```python
from build123d import *

# Parameters (mm, degrees)
F0_R     = 2
F1_DEPTH = 5


with BuildPart() as f1:
    # F0 (on Top) → F1 (new body)
    with BuildSketch(Plane.XY):
        with BuildLine():
            Line((336.332237, -14.014128), (336.332237, 4.985872))
            Line((336.332237, 4.985872), (335.332237, 4.985872))
            Line((335.332237, 4.985872), (335.332237, 5.985872))
            Line((335.332237, 5.985872), (336.332237, 5.985872))
            Line((336.332237, 5.985872), (336.332237, 10.985872))
            Line((336.332237, 10.985872), (295.000411, -0.014128))
            Line((295.000411, -0.014128), (19.999999, -0.007009))
            ThreePointArc((19.999999, -0.007009), (-7.8e-05, -20), (-19.999999, -0.006852))
            Line((-19.999999, -0.006852), (-257.444166, 0.000174))
            ThreePointArc((-257.444166, 0.000174), (-261.686907, -1.75713), (-263.444321, -5.999826))
            Line((-263.444321, -5.999826), (-263.444321, -43.999671))
            ThreePointArc((-263.444321, -43.999671), (-261.686962, -48.242311), (-257.444321, -49.999671))
            Line((-257.444321, -49.999671), (-256, -49.999671))
            ThreePointArc((-256, -49.999671), (-251.757359, -51.75703), (-250, -55.999671))
            Line((-250, -55.999671), (-250, -149.999671))
            ThreePointArc((-250, -149.999671), (-247.071068, -157.070739), (-240, -159.999671))
            Line((-240, -159.999671), (-30.672852, -159.999671))
            ThreePointArc((-30.672852, -159.999671), (-27.473383, -159.474026), (-24.610271, -157.952351))
            Line((-24.610271, -157.952351), (154.720876, -21.24252))
            ThreePointArc((154.720876, -21.24252), (156.438743, -20.329515), (158.358424, -20.014128))
            Line((158.358424, -20.014128), (330.332237, -20.014128))
            ThreePointArc((330.332237, -20.014128), (334.574878, -18.256769), (336.332237, -14.014128))
        make_face()
        with Locations((-50, -120.711)):
            Circle(F0_R, mode=Mode.SUBTRACT)
        with BuildLine():
            Line((-180, -81), (-136, -81))
            ThreePointArc((-136, -81), (-131.757359, -82.757359), (-130, -87))
            Line((-130, -87), (-130, -135))
            ThreePointArc((-130, -135), (-131.757359, -139.242641), (-136, -141))
            Line((-136, -141), (-180, -141))
            ThreePointArc((-180, -141), (-187.071068, -138.071068), (-190, -131))
            Line((-190, -131), (-190, -91))
            ThreePointArc((-190, -91), (-187.071068, -83.928932), (-180, -81))
        make_face(mode=Mode.SUBTRACT)
        with BuildLine():
            Line((-190, -36), (-136, -36))
            ThreePointArc((-136, -36), (-131.757359, -37.757359), (-130, -42))
            Line((-130, -42), (-130, -65))
            ThreePointArc((-130, -65), (-131.757359, -69.242641), (-136, -71))
            Line((-136, -71), (-190, -71))
            Line((-190, -71), (-190, -36))
        make_face(mode=Mode.SUBTRACT)
        Polygon((-155, -21), (-50, -21), (-50, -33), (-95, -33), (-155, -29), (-155, -25), align=None, mode=Mode.SUBTRACT)
    extrude(amount=F1_DEPTH)


solid = f1.part
```
Can you work these out from the model? Positions are in its coordinate system, mm. A direction names the side the tool comes from. Round coordinates to 2 decimals unless told otherwise and drop trailing zeros. Order: outer loops, then holes, each group sorted by start corner. A loop starts at its lowest first (then second) coordinate and runs counter-clockwise, first axis right, second up. Notation, with made-up numbers: (41.5, -18.75) -> (48.5, -18.75) arc R14 ccw to (48.5, 7.25) -> close; hole circle Ø7 at (25, -29). An arc over 180 degrees is marked (long way). Return JSON: item names as keys, results as strings. Group by question number.
1. I need wall thicknesses on line 1 (X direction, y = -122, z = 3.85); line 2 (X direction, y = -121, z = 2.4); line 3 (X direction, y = -138, z = 4.55). Which ranges of each line are inside material? Lowest first, please. Write a range as [from, to].
2. If we section it at B-B, the plane x = -81.5: Write out the boundary of the cut face in (y, z), then the cut area to 3 significant figures.
3. If we section it at D-D, the plane x = 0: Write out the boundary of the cut face in (y, z).
4. We'd pull the mould along X, two halves only. Please class faces 1 (the face through (0, -20, 2)), 2 (the face through (63.8, -90.554, 2.465)), 3 (the face through (-186.99, -138.15, 2.46)), 4 (the face through (-34, -73, 5)): released by +X, released by -X, zero draft, split by the parting line, or undercut.
5. If we section it at A-A, the plane y = -108: Write out the boundary of the cut face in (x, z).
6. Will these pins go through, and if not, where does the flat tip stop? pin 1 (1.5 mm diameter, centred on y = -110.5, z = 2, fed in from +X); pin 2 (1.5 mm diameter, centred on y = -27, z = 2, fed in from +X); pin 3 (0.8 mm diameter, centred on x = 336, z = 1.5, fed in from -Y).
7. If we section it at C-C, the plane z = 1.3: Count the separate pieces of the cut face and the enclosed holes in it, then the cut area to 3 significant figures.
8. Which directions (+Z, -Z, +X, -X, +Y, -Y) give clear straight access to the entire face, cutting with the end or side of a thin tool? Please do faces 5 (the face through (-187.15, -84.01, 2.46)), 6 (the face through (-247.15, -156.99, 2.46)).
Output values:
{
 "1": {"line 1": "[-250, -190], [-130, -51.53], [-48.47, 22.55]", "line 2": "[-250, -190], [-130, -51.98], [-48.02, 23.86]", "line 3": "[-250, -187.14], [-130.8, 1.56]"},
 "2": {"outline": "(-160, 0) -> (-33, 0) -> (-33, 5) -> (-160, 5) -> close; (-21, 0) -> (-0.01, 0) -> (-0.01, 5) -> (-21, 5) -> close", "area": "740 mm²"},
 "3": {"outline": "(-139.19, 0) -> (-20, 0) -> (-20, 5) -> (-139.19, 5) -> close"},
 "4": {"face 1": "undercut", "face 2": "released by +X", "face 3": "undercut", "face 4": "zero draft"},
 "5": {"outline": "(-250, 0) -> (-190, 0) -> (-190, 5) -> (-250, 5) -> close; (-130, 0) -> (40.92, 0) -> (40.92, 5) -> (-130, 5) -> close"},
 "6": {"pin 1": "x = 38.62", "pin 2": "x = 148.15", "pin 3": "y = -16.89"},
 "7": {"separate pieces": "1", "enclosed holes": "4", "area": "49,200 mm²"},
 "8": {"face 5": "+Z, -Z", "face 6": "+Z, -Z, -X, -Y"}
}
